from build123d import *

# Parameters (mm, degrees)
F0_R     = 3.55
F0_R_2   = 11.1
F1_DEPTH = 6.8
F2_R     = 1.5
F3_SIZE  = 0.25


with BuildPart() as f1:
    # F0 (on Top) → F1 (new body)
    with BuildSketch(Plane.XY):
        with BuildLine():
            ThreePointArc((-14, 0), (-12.124355653, 7), (-7, 12.124355653))
            Line((-7, 12.124355653), (-14, 8.0829037687))
            Line((-14, 8.0829037687), (-14, 0))
        make_face()
        with BuildLine():
            ThreePointArc((-7, 12.124355653), (0, 14), (7, 12.124355653))
            Line((7, 12.124355653), (14, 8.0829037687))
            Line((14, 8.0829037687), (14, 35))
            ThreePointArc((14, 35), (11.0454106484, 26.3977384596), (3.4287280559, 21.4263555403))
            ThreePointArc((3.4287280559, 21.4263555403), (3.5195514344, 20.9703556172), (3.55, 20.5063968897))
            ThreePointArc((3.55, 20.5063968897), (-0.4639587275, 16.9868454553), (-3.4287280559, 21.4263555403))
            ThreePointArc((-3.4287280559, 21.4263555403), (-11.0454106484, 26.3977384596), (-14, 35))
            Line((-14, 35), (-14, 8.0829037687))
            Line((-14, 8.0829037687), (-7, 12.124355653))
        make_face()
        with BuildLine():
            ThreePointArc((3.4287280559, 21.4263555403), (11.0454106484, 26.3977384596), (14, 35))
            ThreePointArc((14, 35), (0, 49), (-14, 35))
            ThreePointArc((-14, 35), (-11.0454106484, 26.3977384596), (-3.4287280559, 21.4263555403))
            ThreePointArc((-3.4287280559, 21.4263555403), (0, 24.0563968897), (3.4287280559, 21.4263555403))
        make_face()
        with Locations((0, 29.4450819492)):
            Circle(F0_R, mode=Mode.SUBTRACT)
        with Locations((0, 38.9007553458)):
            Circle(F0_R, mode=Mode.SUBTRACT)
        with BuildLine():
            Line((14, 8.0829037687), (14, 0))
            ThreePointArc((14, 0), (12.124355653, -7), (7, -12.124355653))
            Line((7, -12.124355653), (0, -16.1658075373))
            Line((0, -16.1658075373), (23.3108891325, -29.624355653))
            ThreePointArc((23.3108891325, -29.624355653), (17.3384067843, -22.7644754465), (16.8414041805, -13.6825433692))
            ThreePointArc((16.8414041805, -13.6825433692), (14.6846704631, -8.4781984448), (20.2701322363, -7.7438121711))
            ThreePointArc((20.2701322363, -7.7438121711), (28.3838174327, -3.6332630131), (37.3108891325, -5.375644347))
            Line((37.3108891325, -5.375644347), (14, 8.0829037687))
        make_face()
        with BuildLine():
            ThreePointArc((44.3108891325, -17.5), (42.4352447854, -10.5), (37.3108891325, -5.375644347))
            ThreePointArc((37.3108891325, -5.375644347), (28.3838174327, -3.6332630131), (20.2701322363, -7.7438121711))
            ThreePointArc((20.2701322363, -7.7438121711), (21.0390609624, -8.895222772), (21.3090606466, -10.2531984448))
            ThreePointArc((21.3090606466, -10.2531984448), (19.9206364081, -13.0692400332), (16.8414041805, -13.6825433692))
            ThreePointArc((16.8414041805, -13.6825433692), (17.3384067843, -22.7644754465), (23.3108891325, -29.624355653))
            ThreePointArc((23.3108891325, -29.624355653), (37.3108891325, -29.624355653), (44.3108891325, -17.5))
        make_face()
        with Locations((25.5001889846, -14.7225409746)):
            Circle(F0_R, mode=Mode.SUBTRACT)
        with Locations((33.6890423559, -19.4503776729)):
            Circle(F0_R, mode=Mode.SUBTRACT)
        with BuildLine():
            ThreePointArc((-37.3108891325, -5.375644347), (-42.4352447854, -24.5), (-23.3108891325, -29.624355653))
            ThreePointArc((-23.3108891325, -29.624355653), (-18.1865334795, -24.5), (-16.3108891325, -17.5))
            ThreePointArc((-16.3108891325, -17.5), (-16.4441521456, -15.5729283002), (-16.8414041805, -13.6825433692))
            ThreePointArc((-16.8414041805, -13.6825433692), (-20.83345083, -12.0281984448), (-20.2701322363, -7.7438121711))
            ThreePointArc((-20.2701322363, -7.7438121711), (-28.3838174327, -3.6332630131), (-37.3108891325, -5.375644347))
        make_face()
        with Locations((-33.6890423559, -19.4503776729)):
            Circle(F0_R, mode=Mode.SUBTRACT)
        with Locations((-25.5001889846, -14.7225409746)):
            Circle(F0_R, mode=Mode.SUBTRACT)
        with BuildLine():
            Line((0, -16.1658075373), (-7, -12.124355653))
            ThreePointArc((-7, -12.124355653), (-12.124355653, -7), (-14, 0))
            Line((-14, 0), (-14, 8.0829037687))
            Line((-14, 8.0829037687), (-37.3108891325, -5.375644347))
            ThreePointArc((-37.3108891325, -5.375644347), (-28.3838174327, -3.6332630131), (-20.2701322363, -7.7438121711))
            ThreePointArc((-20.2701322363, -7.7438121711), (-16.4010849737, -6.973198129), (-14.2090606466, -10.2531984448))
            ThreePointArc((-14.2090606466, -10.2531984448), (-14.9430190582, -12.4147742063), (-16.8414041805, -13.6825433692))
            ThreePointArc((-16.8414041805, -13.6825433692), (-16.4441521456, -15.5729283002), (-16.3108891325, -17.5))
            ThreePointArc((-16.3108891325, -17.5), (-18.1865334795, -24.5), (-23.3108891325, -29.624355653))
            Line((-23.3108891325, -29.624355653), (0, -16.1658075373))
        make_face()
        with BuildLine():
            Line((0, -16.1658075373), (7, -12.124355653))
            ThreePointArc((7, -12.124355653), (0, -14), (-7, -12.124355653))
            Line((-7, -12.124355653), (0, -16.1658075373))
        make_face()
        with BuildLine():
            ThreePointArc((7, -12.124355653), (12.124355653, -7), (14, 0))
            ThreePointArc((14, 0), (12.124355653, 7), (7, 12.124355653))
            ThreePointArc((7, 12.124355653), (0, 14), (-7, 12.124355653))
            ThreePointArc((-7, 12.124355653), (-12.124355653, 7), (-14, 0))
            ThreePointArc((-14, 0), (-12.124355653, -7), (-7, -12.124355653))
            ThreePointArc((-7, -12.124355653), (0, -14), (7, -12.124355653))
        make_face()
        Circle(F0_R_2, mode=Mode.SUBTRACT)
        with BuildLine():
            ThreePointArc((7, 12.124355653), (12.124355653, 7), (14, 0))
            Line((14, 0), (14, 8.0829037687))
            Line((14, 8.0829037687), (7, 12.124355653))
        make_face()
    extrude(amount=F1_DEPTH)

    # F2
    f2_edges = [f1.edges().sort_by_distance(p)[0] for p in [
        (-37.310889, -5.375644, 3.4),
        (-23.310889, -29.624356, 3.4),
        (-42.435245, -24.5, 0),
        (-42.435245, -24.5, 6.8),
        (0, -16.165808, 3.4),
        (-11.655445, -22.895082, 0),
        (-11.655445, -22.895082, 6.8),
        (23.310889, -29.624356, 3.4),
        (11.655445, -22.895082, 0),
        (11.655445, -22.895082, 6.8),
        (37.310889, -5.375644, 3.4),
        (42.435245, -24.5, 0),
        (42.435245, -24.5, 6.8),
        (14, 8.082904, 3.4),
        (25.655445, 1.35363, 0),
        (25.655445, 1.35363, 6.8),
        (14, 35, 3.4),
        (14, 21.541452, 0),
        (14, 21.541452, 6.8),
        (-14, 35, 3.4),
        (-14, 8.082904, 3.4),
        (-14, 21.541452, 0),
        (-14, 21.541452, 6.8),
        (-25.655445, 1.35363, 0),
        (-25.655445, 1.35363, 6.8),
    ]]
    fillet(f2_edges, radius=F2_R)

    # F3
    f3_edges = [f1.edges().sort_by_distance(p)[0] for p in [
        (-37.239042, -19.450378, 6.8),
        (-29.050189, -14.722541, 6.8),
        (-18.676717, -6.823854, 6.8),
        (-11.1, 0, 6.8),
        (3.428728, 19.586438, 6.8),
        (-3.55, 29.445082, 6.8),
        (-3.55, 38.900755, 6.8),
        (15.247989, -12.762585, 6.8),
        (21.950189, -14.722541, 6.8),
        (30.139042, -19.450378, 6.8),
    ]]
    chamfer(f3_edges, length=F3_SIZE)


solid = f1.part
Verification items for the finished model (mm, model axes). A direction names the side the tool comes from. Coordinates: 2 decimals unless noted, no trailing zeros. Loops run counter-clockwise (first coordinate to the right, second up) from the corner with the lowest first, then second, coordinate; pieces in that order, holes last. Notation, with made-up numbers: (82.25, 72) -> (128.25, 72) arc R21 cw to (128.25, 107) -> close; hole circle Ø1 at (67.25, 46.25). An arc over 180 degrees is marked (long way). Answer as a JSON object with one key per item and string values. Group by question number.
Item 1: Depth check by flat-ended pin: pin 1 (1 mm diameter, centred on y = 19.5, z = 1.5, fed in from -X); pin 2 (6.5 mm diameter, centred on x = 0, y = 29.45, fed in from +Z); pin 3 (1.9 mm diameter, centred on y = 28, z = 3.5, fed in from +X); pin 4 (2 mm diameter, centred on x = 9.5, z = 3.5, fed in from -Y). Enter the tip coordinate at first touch or a pass-through.
Item 2: Sectioned sample at B-B on z = 3.5. State how many separate pieces and enclosed holes the cut face has, plus the area to 3 significant figures.
Item 3: Tool access check on faces 1 (the flat face through (11.87, -23.02, 3.37)), 2 (the cylindrical face through (-0.77, 35.435, 3.229)), 3 (the flat face through (-14, 22, 3)). Record the directions out of +Z, -Z, +X, -X, +Y, -Y that give a thin tool (end or side, any length) a straight path to the whole face; none if there is none.
Item 4: Mould release check, pull along X, two halves, no side actions. Record for faces 4 (the flat face through (14, 22, 3)), 5 (the cylindrical face through (28.78, -16.08, 3.23)), 6 (the cylindrical face through (-25.97, 0.68, 6.35)): +X half, -X half, draft (parallel to the pull), parting line (faces both ways), or undercut.
Item 5: Scan lines: probe 1 along Y at (x, z) = (0, 2.25); probe 2 along Y at (x, z) = (0, 6.5); probe 3 along X at (y, z) = (9.5, 2.5). Record each from-to range of solid material in increasing order.
Item 6: Sectioned sample at A-A on y = 14.5. Record the boundary of the cut face in (x, z), plus the area to 3 significant figures.
Evaluation:
{
 "1": {"pin 1": "stops at x = -14", "pin 2": "passes through", "pin 3": "stops at x = 14", "pin 4": "stops at y = -22.23"},
 "2": {"separate pieces": "1", "enclosed holes": "10", "area": "2,780 mm²"},
 "3": {"face 1": "+Z, -Z, -Y", "face 2": "+Z, -Z", "face 3": "+Z, -Z, -X, +Y"},
 "4": {"face 4": "+X half", "face 5": "undercut", "face 6": "-X half"},
 "5": {"probe 1": "y = -16.4 to -11.1, 11.1 to 16.96, 24.06 to 25.9, 33 to 35.35, 42.45 to 49", "probe 2": "y = -15.8 to -11.1, 11.1 to 16.96, 24.06 to 25.9, 33 to 35.35, 42.45 to 48.4", "probe 3": "x = -14 to -5.74, 5.74 to 14"},
 "6": {"outline": "(-14, 1.5) arc R1.5 ccw to (-12.5, 0) -> (12.5, 0) arc R1.5 ccw to (14, 1.5) -> (14, 5.3) arc R1.5 ccw to (12.5, 6.8) -> (-12.5, 6.8) arc R1.5 ccw to (-14, 5.3) -> close", "area": "188 mm²"}
}
